Input: part model. Units: mm. Frame: model coordinates. A direction names the side the tool comes from. Coordinates: 2 decimals unless noted, no trailing zeros. Loops run counter-clockwise (first coordinate to the right, second up) from the corner with the lowest first, then second, coordinate; pieces in that order, holes last.
(1) Section C-C, the plane y = 10. Return loops of the section in (x, z), then the cut area to 3 significant figures.
(2) Section D-D, the plane y = 1.5. Return loops of the section in (x, z), then the cut area to 3 significant figures.
(3) Set-up query: faces 4 (the face through (40, -24, 32)), 5 (the face through (-33, -25, 29)), 6 (the face through (1, -23, 18)), 7 (the face through (-49, 3, 30)). Return all of +Z, -Z, +X, -X, +Y, -Y with unobstructed straight access to the full face (end or side cutting, diameter ignored); none if empty.
(4) Line query: L1, parallel to Y at x = -17, z = 28; L2, parallel to Z at x = 41.5, y = 21; L3, parallel to X at y = 13, z = 6.5. Output: solid intervals per line, ascending.
(5) Section A-A, the plane x = -16. Return loops of the section in (y, z), then the cut area to 3 significant figures.
(6) Section B-B, the plane z = 27. Return loops of the section in (x, y), then the cut area to 3 significant figures.
(7) Mould query, pull axis Y, two halves, no side actions, for faces 1 (the face through (-49, 0, 29)), 2 (the face through (-1, -26, 16)), 3 (the face through (30, 24, 30)). Classes: released by +Y, released by -Y, zero draft, split by the parting line, or undercut.
(8) Contact query for flat-ended pins moving along their axis: P1, Ø1.5, axis at x = -33.5, y = 24.5, coming from the +Z side; P2, Ø8, axis at y = 7.5, z = 25.5, coming from the +X side; P3, Ø23, axis at x = 23, y = -5.5, coming from the +Z side. Output: stop coordinate, or through.
```python
from build123d import *

# Parameters (mm, degrees)
F0_W     = 100
F0_H     = 52
F1_DEPTH = 32
F2_W     = 97
F2_H     = 46
F3_DEPTH = 29
F4_W     = 6
F4_H     = 3
F5_DEPTH = 52.001
F6_W     = 6
F6_H     = 3
F7_DEPTH = 52.001
F8_W     = 6
F8_H     = 3
F9_DEPTH = 100.001


with BuildPart() as f1:
    # F0 (on Top) → F1 (new body)
    with BuildSketch(Plane.XY):
        Rectangle(F0_W, F0_H)
    extrude(amount=F1_DEPTH)

    # F2 (on face) → F3 (cut)
    with BuildSketch(Plane.XY.offset(32)):
        with Locations((1.5, 0)):
            Rectangle(F2_W, F2_H)
    extrude(amount=-F3_DEPTH, mode=Mode.SUBTRACT)

    # F4 (on face) → F5 (cut, through all)
    with BuildSketch(Plane.XZ.offset(26)):
        with Locations((-33, 30.5)):
            Rectangle(F4_W, F4_H)
    extrude(amount=-F5_DEPTH, mode=Mode.SUBTRACT)

    # F6 (on face) → F7 (cut, through all)
    with BuildSketch(Plane.XZ.offset(26)):
        with Locations((27, 30.5)):
            Rectangle(F6_W, F6_H)
    extrude(amount=-F7_DEPTH, mode=Mode.SUBTRACT)

    # F8 (on face) → F9 (cut, through all)
    with BuildSketch(Plane(origin=(-50, 0, 0), x_dir=(0, -1, 0), z_dir=(-1, 0, 0))):
        with Locations((0, 30.5)):
            Rectangle(F8_W, F8_H)
    extrude(amount=-F9_DEPTH, mode=Mode.SUBTRACT)


solid = f1.part
```
Report:
1. outline: (-50, 0) - (50, 0) - (50, 3) - (-47, 3) - (-47, 32) - (-50, 32) - close
1. area: 387 mm2
2. outline: (-50, 0) - (50, 0) - (50, 3) - (-47, 3) - (-47, 29) - (-50, 29) - close
2. area: 378 mm2
3. face 4: +Z, +X, -X, +Y, -Y
3. face 5: +Z, +Y, -Y
3. face 6: +Z, +X
3. face 7: +Z, +X, -X
4. L1: y = -26 to -23, 23 to 26
4. L2: z = 0 to 3
4. L3: x = -50 to -47
5. outline: (-26, 0) - (26, 0) - (26, 32) - (23, 32) - (23, 3) - (-23, 3) - (-23, 32) - (-26, 32) - close
5. area: 330 mm2
6. outline: (-50, -26) - (50, -26) - (50, -23) - (-47, -23) - (-47, 23) - (50, 23) - (50, 26) - (-50, 26) - close
6. area: 738 mm2
7. face 1: undercut
7. face 2: released by -Y
7. face 3: zero draft
8. P1: stops at z = 29
8. P2: stops at x = -47
8. P3: stops at z = 3
